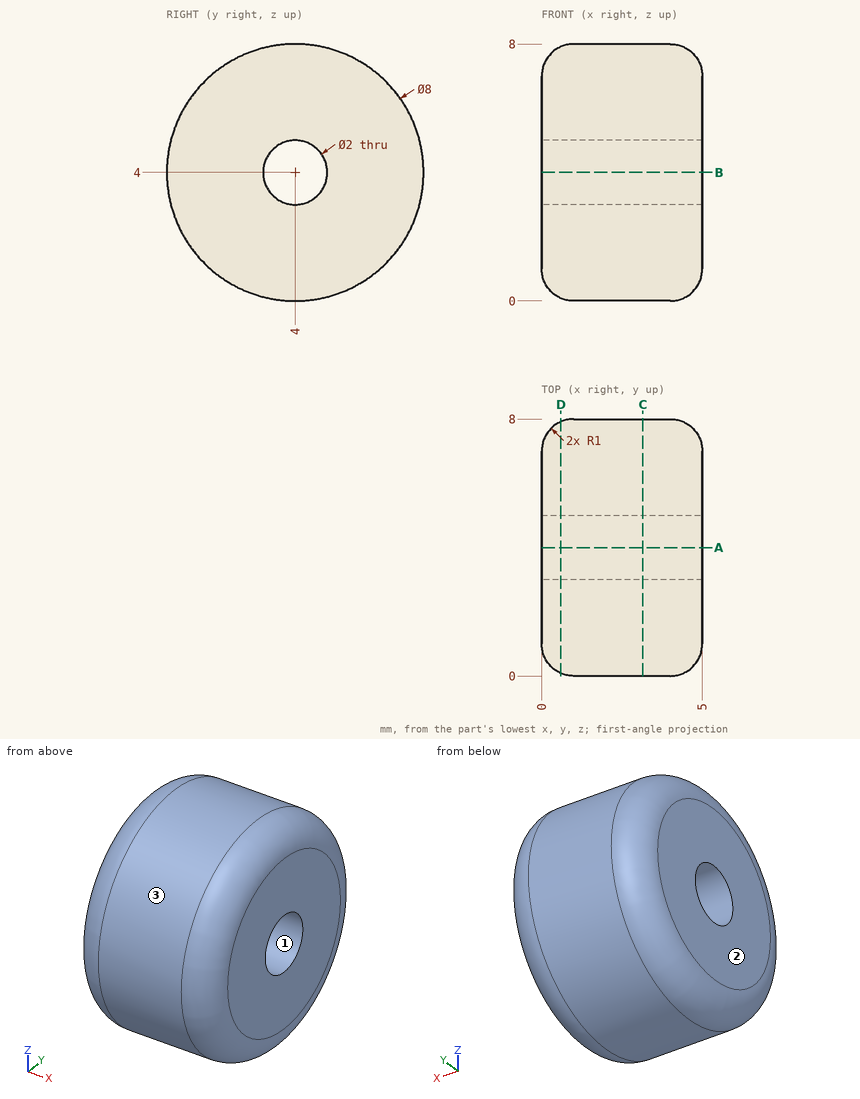
Check sheet for the drawn part. Datum: minimum x, y, z corner. Units: mm. Coordinates: 2 decimals unless noted, no trailing zeros. Order: outer loops, then holes, each group sorted by start corner. A loop starts at its lowest first (then second) coordinate and runs counter-clockwise, first axis right, second up. Notation, with made-up numbers: (25.5, 57) -> (44.5, 57) arc R13 cw to (44.5, 73) -> close; hole circle Ø5 at (29.25, 32.25). An arc over 180 degrees is marked (long way). Use a Markdown table: item, result. Add a question column.
1. Material ranges on L1, parallel to Z at x = 3, y = 4; L2, parallel to X at y = 0.5, z = 4.75 (3 decimals); L3, parallel to Z at x = 4.3, y = 6.25, recorded low to high.
2. Cross-section at D-D (x = 0.6). Enter the section's corners in (y, z).
3. Cross-section at C-C (x = 3.15). Enter the section's corners in (y, z), and give its area (3 significant figures).
4. Go/stop test with flat-tipped pins: pin 1 Ø1.2 at (y, z) = (4, 4) entering from -X; pin 2 Ø1 at (x, y) = (4.5, 3.5) entering from -Z. Record where each tip stops, or that it passes through.
5. Mould release check, pull along Z, two halves, no side actions. Record for the marked faces 1, 2 and 3: pulls with the +Z half, pulls with the -Z half, needs draft (parallel to the pull), parting line crosses it, or undercut.
6. Cross-section at A-A (y = 4). Enter the section's corners in (x, z), and give its area (3 significant figures).
Filled sheet:
| question | item | result |
|---|---|---|
| 1 | L1 | 0 to 3, 5 to 8 |
| 1 | L2 | 0.185 to 4.815 |
| 1 | L3 | 0.75 to 7.25 |
| 2 | outline | circle Ø7.83 at (4, 4); hole circle Ø2 at (4, 4) |
| 3 | outline | circle Ø8 at (4, 4); hole circle Ø2 at (4, 4) |
| 3 | area | 47.1 mm2 |
| 4 | pin 1 | through |
| 4 | pin 2 | z = 0.01 |
| 5 | face 1 | undercut |
| 5 | face 2 | needs draft |
| 5 | face 3 | parting line crosses it |
| 6 | outline | (0, 1) arc R1 ccw to (1, 0) -> (4, 0) arc R1 ccw to (5, 1) -> (5, 3) -> (0, 3) -> close; (0, 5) -> (5, 5) -> (5, 7) arc R1 ccw to (4, 8) -> (1, 8) arc R1 ccw to (0, 7) -> close |
| 6 | area | 29.1 mm2 |
